```python
from build123d import *

# Parameters (mm, degrees)
BOSS_EXTRUDE1_DEPTH = 22.225
SKETCH2_R           = 3.302
CUT_EXTRUDE1_DEPTH  = 59.630138368
BOSS_EXTRUDE2_DEPTH = 3.175
SKETCH4_R           = 1.000000032
CUT_EXTRUDE2_DEPTH  = 56.901643536


with BuildPart() as part:
    # Sketch1 → Boss-Extrude1 (new, symmetric)
    with BuildSketch(Plane.XY):
        Polygon((0, 0), (0, 50.8), (3.175, 50.8), (3.175, 3.175), (19.05, 3.175), (19.05, 0), align=None)
    extrude(amount=BOSS_EXTRUDE1_DEPTH, both=True)

    # Sketch2 → Cut-Extrude1 (cut, through all)
    with BuildSketch(Plane.ZY):
        with Locations((-6.35, 39.9542)):
            Circle(SKETCH2_R)
    extrude(amount=-CUT_EXTRUDE1_DEPTH, mode=Mode.SUBTRACT)

    # Sketch3 → Boss-Extrude2 (add)
    with BuildSketch(Plane.XY.offset(22.225)):
        Polygon((3.175, 50.8), (19.05, 3.175), (3.175, 3.175), align=None)
    boss_extrude2 = extrude(amount=-BOSS_EXTRUDE2_DEPTH)

    # Mirror1: Boss-Extrude2 across plane
    add(boss_extrude2.mirror(Plane.XY))

    # Sketch4 → Cut-Extrude2 (cut, through all)
    with BuildSketch(Plane(origin=(0, 3.175, 0), x_dir=(1, 0, 0), z_dir=(0, 1, 0))):
        with Locations(Location((6.35, 12.7, 0), (0, 0, 180))):
            Circle(SKETCH4_R)
        with Locations(Location((15.24, 12.7, 0), (0, 0, 180))):
            Circle(SKETCH4_R)
        with Locations((15.24, -12.7)):
            Circle(SKETCH4_R)
        with Locations((6.35, -12.7)):
            Circle(SKETCH4_R)
    extrude(amount=-CUT_EXTRUDE2_DEPTH, mode=Mode.SUBTRACT)


solid = part.part
```
Input: part model. Units: mm. Frame: model coordinates. A direction names the side the tool comes from. Round coordinates to 2 decimals unless told otherwise and drop trailing zeros. Order: outer loops, then holes, each group sorted by start corner. A loop starts at its lowest first (then second) coordinate and runs counter-clockwise, first axis right, second up. Notation, with made-up numbers: (20, -0.75) - (71, -0.75) arc R20 ccw to (71, 27.25) - close; hole circle Ø8 at (66, -14.5). An arc over 180 degrees is marked (long way). Answer in a Markdown table with one row per item.
Item 1: Reachability of faces 4 (the flat face through (3.175, 27, 0)), 5 (the cylindrical face through (5.81, 1.61, -11.86)) from +Z, -Z, +X, -X, +Y, -Y: full face, straight path, thin tool, end or side. Return the list, or none.
Model answer:
| item | result |
|---|---|
| face 4 | +X, +Y |
| face 5 | +Y, -Y |
Item 2: Section query D-D (x = 12). Return the cut outline in (y, z) (3 decimals), then the cut area to 3 significant figures.
Model answer:
| item | result |
|---|---|
| outline | (0, -22.225) - (24.325, -22.225) - (24.325, -19.05) - (3.175, -19.05) - (3.175, 19.05) - (24.325, 19.05) - (24.325, 22.225) - (0, 22.225) - close |
| area | 275 mm² |
Item 3: Section query A-A (z = -6.35). Return the cut outline in (x, y) (3 decimals), then the cut area to 3 significant figures.
Model answer:
| item | result |
|---|---|
| outline | (0, 0) - (19.05, 0) - (19.05, 3.175) - (3.175, 3.175) - (3.175, 36.652) - (0, 36.652) - close; (0, 43.256) - (3.175, 43.256) - (3.175, 50.8) - (0, 50.8) - close |
| area | 191 mm² |
Item 4: Line query: line 1 (Z direction, x = 6.35, y = 1.9) (3 decimals); line 2 (Y direction, x = 1.1, z = -6.35); line 3 (Z direction, x = 4.25, y = 17.5) (3 decimals). Output: solid intervals per line, ascending.
Model answer:
| item | result |
|---|---|
| line 1 | z = -22.225 to -13.7, -11.7 to 11.7, 13.7 to 22.225 |
| line 2 | y = 0 to 36.65, 43.26 to 50.8 |
| line 3 | z = -22.225 to -19.05, 19.05 to 22.225 |
Item 5: Section query B-B (z = -12.7). Return the cut outline in (x, y) (3 decimals), then the cut area to 3 significant figures.
Model answer:
| item | result |
|---|---|
| outline | (0, 0) - (5.35, 0) - (5.35, 3.175) - (3.175, 3.175) - (3.175, 50.8) - (0, 50.8) - close; (7.35, 0) - (14.24, 0) - (14.24, 3.175) - (7.35, 3.175) - close; (16.24, 0) - (19.05, 0) - (19.05, 3.175) - (16.24, 3.175) - close |
| area | 199 mm² |
Item 6: Section query C-C (x = 6.35). Return the cut outline in (y, z) (3 decimals), then the cut area to 3 significant figures.
Model answer:
| item | result |
|---|---|
| outline | (0, -22.225) - (41.275, -22.225) - (41.275, -19.05) - (3.175, -19.05) - (3.175, -13.7) - (0, -13.7) - close; (0, -11.7) - (3.175, -11.7) - (3.175, 11.7) - (0, 11.7) - close; (0, 13.7) - (3.175, 13.7) - (3.175, 19.05) - (41.275, 19.05) - (41.275, 22.225) - (0, 22.225) - close |
| area | 370 mm² |
Item 7: Pin query (flat end, axial travel): pin 1 (12 mm diameter, centred on y = 30.5, z = 0.5, fed in from +X) (3 decimals); pin 2 (2.5 mm diameter, centred on x = 6.35, z = 12.7, fed in from +Y) (3 decimals). Return the tip coordinate at first contact, or that it passes through.
Model answer:
| item | result |
|---|---|
| pin 1 | stops at x = 3.175 |
| pin 2 | stops at y = 3.175 |
Item 8: Mould query, pull axis Z, two halves, no side actions, for faces 1 (the flat face through (11, 27.32, -20.66)), 2 (the flat face through (8, 20, 22.225)), 3 (the cylindrical face through (1.565, 42.738, -4.575)). Classes: released by +Z, released by -Z, zero draft, split by the parting line, or undercut.
Model answer:
| item | result |
|---|---|
| face 1 | zero draft |
| face 2 | released by +Z |
| face 3 | undercut |
